Autodesk Inventor part; units mm, degrees
ref_plane "YZ Plane" through (0, 0, 0) normal (1, 0, 0) x (0, 1, 0)
ref_plane "XZ Plane" through (0, 0, 0) normal (0, 1, 0) x (-1, 0, 0)
ref_plane "XY Plane" through (0, 0, 0) normal (0, 0, 1) x (1, 0, 0)
sketch "Sketch1" plane through (0, 0, 0) normal (1, 0, 0) x (0, 1, 0)
  line L0 (-12, 32.5) -> (12, 32.5)
  line L1 (15, 29.5) -> (15, -29.5)
  line L2 (12, -32.5) -> (-12, -32.5)
  line L3 (-15, -29.5) -> (-15, 29.5)
  line L4 (-15, 32.5) -> (15, -32.5) construction
  line L5 (15, 32.5) -> (-15, -32.5) construction
  arc A0 (-12, 32.5) -> (-15, 29.5) centre (-12, 29.5) ccw
  arc A1 (15, 29.5) -> (12, 32.5) centre (12, 29.5) ccw
  arc A2 (12, -32.5) -> (15, -29.5) centre (12, -29.5) ccw
  arc A3 (-15, -29.5) -> (-12, -32.5) centre (-12, -29.5) ccw
  point P0 (0, 0)
  dimension "d0" = 30
  dimension "d1" = 65
  dimension "d22" = 3
extrude "Extrusion1" add sketch "Sketch1" along normal blind 1.5
fillet "Fillet1" [suppressed]
sketch "Sketch2" plane through (1.5, 0, 0) normal (1, 0, 0) x (0, 0, -1)
  line L0 (29.5, 15) -> (-29.5, 15)
  line L1 (-32.5, 12) -> (-32.5, -12)
  arc A0 (-32.5, -12) -> (-29.5, -15) centre (-29.5, -12) ccw
  point P0 (0, 0)
  point P1 (-29.5, 11)
  point P2 (32, 15)
  point P3 (-32, 15)
  point P4 (-33, 14)
  point P5 (-33, -14)
  point P6 (28.5, 11)
  point P7 (28.5, -12)
  dimension "d5" = 4
  dimension "d6" = 3
  dimension "d9" = 58
  dimension "d12" = 23
hole "Hole1" at (1.5, 11, 29.5) at (1.5, 11, -28.5) at (1.5, -12, 29.5) at (1.5, -12, -28.5) direction (-1, 0, 0) diameter 2.75 end through all
properties part number "RPI_Zero"
Check sheet for the modelled part. Datum: model origin and axes. Units: mm. Round coordinates to 2 decimals unless told otherwise and drop trailing zeros. Loops run counter-clockwise (first coordinate to the right, second up) from the corner with the lowest first, then second, coordinate; pieces in that order, holes last. Notation, with made-up numbers: (55, -37.5) - (110, -37.5) arc R15 ccw to (110, -23.5) - close; hole circle Ø4 at (57.5, 32.25). An arc over 180 degrees is marked (long way). Answer as a JSON object with one key per item and string values. Group by question number.
Q1. Sectioned sample at C-C, the plane x = 0.3. Enter the section's corners in (y, z) (3 decimals).
Q2. Scan lines: line 1 along Z through (x, y) = (0.9, 11) (3 decimals); line 2 along Y through (x, z) = (1.15, 29.5) (3 decimals); line 3 along Z through (x, y) = (1.35, 12). Record each from-to range of solid material in increasing order. Write a range as [from, to].
Q3. Sectioned sample at B-B, the plane y = 11. Enter the section's corners in (x, z) (3 decimals), plus the area to 4 significant figures.
Q4. Mould release check, pull along Z, two halves, no side actions. Record for faces 1 (the face through (0.74, -12.06, 30.874)), 2 (the face through (0, 0, 0)), 3 (the face through (0.74, -12.06, -27.126)), 4 (the face through (1, 0, -32.5)): released by +Z, released by -Z, zero draft, split by the parting line, or undercut.
Q5. Gauge pin test, flat ends, axial feed: P1, Ø2, axis at y = 11, z = 29.5, coming from the +X side; P2, Ø12, axis at y = 0.5, z = 24, coming from the -X side. Record the tip position at first contact, or that the pin passes through.
Q6. Sectioned sample at A-A, the plane z = -28.5. Enter the section's corners in (x, y) (3 decimals).
Solution:
{
 "1": {"outline": "(-15, -29.5) arc R3 ccw to (-12, -32.5) - (12, -32.5) arc R3 ccw to (15, -29.5) - (15, 29.5) arc R3 ccw to (12, 32.5) - (-12, 32.5) arc R3 ccw to (-15, 29.5) - close; hole circle Ø2.75 at (-12, -28.5); hole circle Ø2.75 at (-12, 29.5); hole circle Ø2.75 at (11, -28.5); hole circle Ø2.75 at (11, 29.5)"},
 "2": {"line 1": "z = [-32.5, -29.875], [-27.125, 28.125], [30.875, 32.5]", "line 2": "y = [-15, -13.375], [-10.625, 9.625], [12.375, 15]", "line 3": "z = [-32.5, -29.44], [-27.56, 28.56], [30.44, 32.5]"},
 "3": {"outline": "(0, -32.5) - (1.5, -32.5) - (1.5, -29.875) - (0, -29.875) - close; (0, -27.125) - (1.5, -27.125) - (1.5, 28.125) - (0, 28.125) - close; (0, 30.875) - (1.5, 30.875) - (1.5, 32.5) - (0, 32.5) - close", "area": "89.25 mm²"},
 "4": {"face 1": "undercut", "face 2": "zero draft", "face 3": "undercut", "face 4": "released by -Z"},
 "5": {"P1": "passes through", "P2": "stops at x = 0"},
 "6": {"outline": "(0, -15) - (1.5, -15) - (1.5, -13.375) - (0, -13.375) - close; (0, -10.625) - (1.5, -10.625) - (1.5, 9.625) - (0, 9.625) - close; (0, 12.375) - (1.5, 12.375) - (1.5, 15) - (0, 15) - close"}
}
